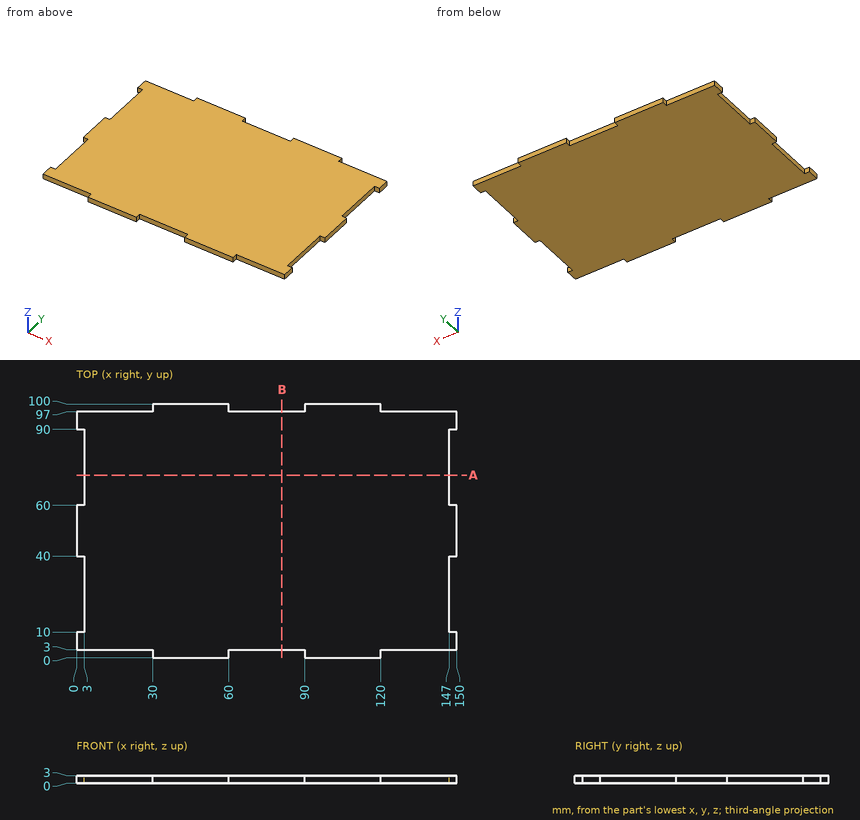
Job drawing, mm, ordinate dimensions from the low corner. One solid piece. Give positions to 0.01 mm unless a question says otherwise; leave off trailing zeros. Loops run counter-clockwise (first coordinate to the right, second up) from the corner with the lowest first, then second, coordinate; pieces in that order, holes last. Notation, with made-up numbers: M 26.5,-32.75 L 46.5,-32.75 A21 ccw 46.5,-11.75 Z; hole C 20,-36 d7. An arc over 180 degrees is marked long. Put each result on its own line as item: value. Start each with the question number.
1) Saw through at B-B (x = 81). List the corners of the cut face in (y, z), then the cut area to 3 significant figures.
2) Flat gauge pins, fed straight in: pin 1 (1.5 mm diameter, centred on y = 1, z = 1.5, fed in from -X); pin 2 (0.9 mm diameter, centred on y = 98.5, z = 1, fed in from +X); pin 3 (1.5 mm diameter, centred on x = 82.5, z = 1.5, fed in from +Y); pin 4 (8 mm diameter, centred on x = 50.5, y = 60, fed in from -Z). Where does each tip first touch, or does it go through?
3) Probe probe 1 along Y at (x, z) = (130.5, 1.65); probe 2 along X at (y, z) = (84.5, 2.3). List the from-to ranges inside material, lowest first.
4) Saw through at A-A (y = 72). List the corners of the cut face in (x, z).
Numbers:
1. outline: M 3,0 L 97,0 L 97,3 L 3,3 Z
1. area: 282 mm^2
2. pin 1: x = 30
2. pin 2: x = 120
2. pin 3: y = 97
2. pin 4: z = 0
3. probe 1: 3 to 97
3. probe 2: 3 to 147
4. outline: M 3,0 L 147,0 L 147,3 L 3,3 Z
